from build123d import *

# Parameters (mm, degrees)
EXTRUDE_1_DEPTH     = 40
EXTRUDE_2_DEPTH     = 10
CUT_EXTRUDE_1_REACH = 53.713
CUT_EXTRUDE_2_REACH = 53.713


with BuildPart() as part:
    # 스케치1 → 보스-돌출1 (new body)
    with BuildSketch(Plane.XY):
        with BuildLine():
            ThreePointArc((8, 0), (0, 8), (-8, 0))
            Line((-8, 0), (-4, 0))
            ThreePointArc((-4, 0), (0, 4), (4, 0))
            Line((4, 0), (8, 0))
        make_face()
        with BuildLine():
            ThreePointArc((4, 0), (0, 4), (-4, 0))
            Line((-4, 0), (4, 0))
        make_face()
    extrude(amount=EXTRUDE_1_DEPTH)

    # 스케치6 → 보스-돌출2 (add)
    with BuildSketch(Plane.XY.offset(40)):
        Polygon((0, 0), (2.5, 0), (2.5, 7.599342077), (-2.5, 7.599342077), (-2.5, 0), align=None)
    extrude(amount=EXTRUDE_2_DEPTH)

    # 스케치8 → 컷-돌출1 (cut, up to next)
    with BuildSketch(Plane(origin=(2.5, 0, 0), x_dir=(0, 0, -1), z_dir=(1, 0, 0)), mode=Mode.PRIVATE) as cut_extrude_1_sk1:
        with BuildLine():
            Line((-50, 7.599342077), (-50, 3.799671038))
            ThreePointArc((-50, 3.799671038), (-48.887102119, 6.486444196), (-46.200328962, 7.599342077))
            Line((-46.200328962, 7.599342077), (-50, 7.599342077))
        make_face()
    cut_extrude_1_tool1 = extrude(cut_extrude_1_sk1.sketch, amount=-CUT_EXTRUDE_1_REACH, mode=Mode.PRIVATE) & part.part
    # 스케치8 → 컷-돌출1 (cut, up to next)
    with BuildSketch(Plane(origin=(2.5, 0, 0), x_dir=(0, 0, -1), z_dir=(1, 0, 0)), mode=Mode.PRIVATE) as cut_extrude_1_sk2:
        with BuildLine():
            ThreePointArc((-46.200328962, 0), (-48.887102119, 1.112897881), (-50, 3.799671038))
            Line((-50, 3.799671038), (-50, 0))
            Line((-50, 0), (-46.200328962, 0))
        make_face()
    cut_extrude_1_tool2 = extrude(cut_extrude_1_sk2.sketch, amount=-CUT_EXTRUDE_1_REACH, mode=Mode.PRIVATE) & part.part
    add(cut_extrude_1_tool1.solids().sort_by_distance((2.5, 6.750617, 49.151275))[0], mode=Mode.SUBTRACT)
    add(cut_extrude_1_tool2.solids().sort_by_distance((2.5, 0.848725, 49.151275))[0], mode=Mode.SUBTRACT)

    # 스케치8<4> → 컷-돌출2 (cut, up to next)
    with BuildSketch(Plane(origin=(2.5, 0, 0), x_dir=(0, 0, -1), z_dir=(1, 0, 0)), mode=Mode.PRIVATE) as cut_extrude_2_sk1:
        with BuildLine():
            ThreePointArc((-48.200328962, 3.799671038), (-46.200328962, 1.799671038), (-44.200328962, 3.799671038))
            Line((-44.200328962, 3.799671038), (-48.200328962, 3.799671038))
        make_face()
    cut_extrude_2_tool1 = extrude(cut_extrude_2_sk1.sketch, amount=-CUT_EXTRUDE_2_REACH, mode=Mode.PRIVATE) & part.part
    # 스케치8<4> → 컷-돌출2 (cut, up to next)
    with BuildSketch(Plane(origin=(2.5, 0, 0), x_dir=(0, 0, -1), z_dir=(1, 0, 0)), mode=Mode.PRIVATE) as cut_extrude_2_sk2:
        with BuildLine():
            Line((-48.200328962, 3.799671038), (-44.200328962, 3.799671038))
            ThreePointArc((-44.200328962, 3.799671038), (-46.200328962, 5.799671038), (-48.200328962, 3.799671038))
        make_face()
    cut_extrude_2_tool2 = extrude(cut_extrude_2_sk2.sketch, amount=-CUT_EXTRUDE_2_REACH, mode=Mode.PRIVATE) & part.part
    # 스케치8<4> → 컷-돌출2 (cut, up to next)
    with BuildSketch(Plane(origin=(2.5, 0, 0), x_dir=(0, 0, -1), z_dir=(1, 0, 0)), mode=Mode.PRIVATE) as cut_extrude_2_sk3:
        with BuildLine():
            ThreePointArc((-48.200328962, 3.799671038), (-46.200328962, 1.799671038), (-44.200328962, 3.799671038))
            Line((-44.200328962, 3.799671038), (-48.200328962, 3.799671038))
        make_face()
    cut_extrude_2_tool3 = extrude(cut_extrude_2_sk3.sketch, amount=-CUT_EXTRUDE_2_REACH, mode=Mode.PRIVATE) & part.part
    # 스케치8<4> → 컷-돌출2 (cut, up to next)
    with BuildSketch(Plane(origin=(2.5, 0, 0), x_dir=(0, 0, -1), z_dir=(1, 0, 0)), mode=Mode.PRIVATE) as cut_extrude_2_sk4:
        with BuildLine():
            Line((-48.200328962, 3.799671038), (-44.200328962, 3.799671038))
            ThreePointArc((-44.200328962, 3.799671038), (-46.200328962, 5.799671038), (-48.200328962, 3.799671038))
        make_face()
    cut_extrude_2_tool4 = extrude(cut_extrude_2_sk4.sketch, amount=-CUT_EXTRUDE_2_REACH, mode=Mode.PRIVATE) & part.part
    add(cut_extrude_2_tool1.solids().sort_by_distance((2.5, 2.950845, 46.200329))[0], mode=Mode.SUBTRACT)
    add(cut_extrude_2_tool2.solids().sort_by_distance((2.5, 4.648497, 46.200329))[0], mode=Mode.SUBTRACT)
    add(cut_extrude_2_tool3.solids().sort_by_distance((2.5, 2.950845, 46.200329))[0], mode=Mode.SUBTRACT)
    add(cut_extrude_2_tool4.solids().sort_by_distance((2.5, 4.648497, 46.200329))[0], mode=Mode.SUBTRACT)


solid = part.part
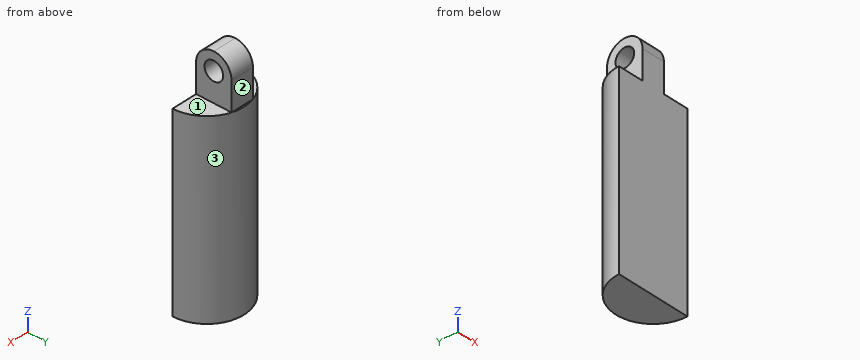
Here's how the part is built. I have some questions about the finished solid (model axes, mm). Face numbers are marked on the shaded views. A direction names the side the tool comes from. Round coordinates to 2 decimals unless told otherwise and drop trailing zeros. Write each loop counter-clockwise with the first axis right and the second up, starting at its lowest first coordinate (ties: lowest second). Pieces come first, ordered by that corner, then holes. Notation, with made-up numbers: (65.25, -33) -> (101.25, -33) arc R9 cw to (101.25, -28) -> close; hole circle Ø4 at (18.25, -35.5). An arc over 180 degrees is marked (long way). One line per item, written item: value.
1) If I drill on line 1 (Y direction, x = 5.5, z = 24); line 2 (X direction, y = 6, z = 44); line 3 (Z direction, x = 5, y = 6), over which ranges is the centre line in solid material (lowest first)? Write a range as [from, to].
Filled sheet:
line 1: y = [0, 5.81]
line 2: x = [-2.5, 2.5]
line 3: z = [0, 40]
2) Suppose I cut it at C-C on y = 7. List the corners of the cut face in (x, z) for me, plus the area to 3 significant figures.
Filled sheet:
outline: (-3.87, 0) -> (3.87, 0) -> (3.87, 40) -> (2.5, 40) -> (2.5, 48.25) -> (-2.5, 48.25) -> (-2.5, 40) -> (-3.87, 40) -> close
area: 351 mm2
3) For the marked faces 1, 2 and 3, which set-ups out of +Z, -Z, +X, -X, +Y, -Y let a thin tool reach every point of the face, with its end or its side?
Filled sheet:
face 1: +Z, +X, +Y, -Y
face 2: +Z, +X, -X, +Y
face 3: +Z, -Z, +Y
4) Suppose I cut it at B-B on y = 4.5. List the corners of the cut face in (x, z) for me, plus the area to 3 significant figures.
Filled sheet:
outline: (-6.61, 0) -> (6.61, 0) -> (6.61, 40) -> (2.5, 40) -> (2.5, 44.33) -> (-2.5, 44.33) -> (-2.5, 40) -> (-6.61, 40) -> close; (-2.5, 48.07) -> (2.5, 48.07) -> (2.5, 49.93) -> (-2.5, 49.93) -> close
area: 560 mm2
5) Suppose I cut it at D-D on z = 17. List the corners of the cut face in (x, y) for me.
Filled sheet:
outline: (-8, 0) -> (8, 0) arc R8 ccw to start
6) I'm going to push flat-ended pins straight in: pin 1 Ø3 at (x, y) = (6, 3) entering from +Z; pin 2 Ø2.5 at (y, z) = (3, 46) entering from +X; pin 3 Ø4.5 at (y, z) = (3.8, 46.2) entering from -X; pin 4 Ø1 at (x, y) = (-5.5, 7) entering from +Z. Where does each tip first touch, or does it pass through?
Filled sheet:
pin 1: stops at z = 40
pin 2: stops at x = 2.5
pin 3: stops at x = -2.5
pin 4: passes through
7) Suppose I cut it at A-A on x = 0. List the corners of the cut face in (y, z) for me.
Filled sheet:
outline: (0, 0) -> (8, 0) -> (8, 40) -> (7.6, 40) -> (7.6, 46.2) arc R3.8 ccw to (0, 46.2) -> close; hole circle Ø4 at (3.8, 46.2)
